from build123d import *

# Parameters (mm, degrees)
SKETCH1_R           = 1.4605
BOSS_EXTRUDE1_DEPTH = 3.175
CUT_EXTRUDE1_REACH  = 105.107
CUT_EXTRUDE2_REACH  = 105.107
SKETCH4_W           = 25.4
SKETCH4_H           = 7.62
CUT_EXTRUDE3_DEPTH  = 36.774302562


with BuildPart() as part:
    # Sketch1 → Boss-Extrude1 (new body)
    with BuildSketch(Plane.XY):
        with BuildLine():
            Line((0, 7.62), (0, 25.4))
            ThreePointArc((0, 25.4), (-17.960512242, -17.960512242), (25.4, 0))
            Line((25.4, 0), (16.51, 0))
            Line((16.51, 0), (16.51, -3.175))
            Line((16.51, -3.175), (13.589, -3.175))
            Line((13.589, -3.175), (13.589, -9.779))
            Line((13.589, -9.779), (15.494, -9.779))
            Line((15.494, -9.779), (15.494, -12.827))
            Line((15.494, -12.827), (13.589, -12.827))
            Line((13.589, -12.827), (10.541, -12.827))
            Line((10.541, -12.827), (8.636, -12.827))
            Line((8.636, -12.827), (8.636, -9.779))
            Line((8.636, -9.779), (10.541, -9.779))
            Line((10.541, -9.779), (10.541, -3.175))
            Line((10.541, -3.175), (7.62, -3.175))
            Line((7.62, -3.175), (7.62, 0))
            ThreePointArc((7.62, 0), (5.388153673, 5.388153673), (0, 7.62))
        make_face()
        with Locations((20.955, -1.5875)):
            Circle(SKETCH1_R, mode=Mode.SUBTRACT)
        Polygon((3.175, 1.833087105), (3.175, -1.833087105), (0, -3.666174209), (-3.175, -1.833087105), (-3.175, 1.833087105), (0, 3.666174209), align=None, mode=Mode.SUBTRACT)
    extrude(amount=BOSS_EXTRUDE1_DEPTH)

    # Sketch2 → Cut-Extrude1 (cut, up to next)
    with BuildSketch(Plane(origin=(0, 0, -93.472), x_dir=(-1, 0, 0), z_dir=(0, 0, -1)), mode=Mode.PRIVATE) as cut_extrude1_sk1:
        Polygon((-4.538711403, -7.782479393), (27.834438784, -7.782479393), (16.089332095, -38.12601526), (-4.538711403, -36.427419359), align=None)
    cut_extrude1_tool1 = extrude(cut_extrude1_sk1.sketch, amount=-CUT_EXTRUDE1_REACH, mode=Mode.PRIVATE) & part.part
    add(cut_extrude1_tool1.solids().sort_by_distance((-9.075281, -21.483297, -93.472))[0], mode=Mode.SUBTRACT)

    # Sketch3 → Cut-Extrude2 (cut, up to next)
    with BuildSketch(Plane(origin=(0, 0, -93.472), x_dir=(-1, 0, 0), z_dir=(0, 0, -1)), mode=Mode.PRIVATE) as cut_extrude2_sk1:
        Polygon((8.30871298, -7.782479393), (8.30871298, 15.866972004), (0, 15.866972004), (0, 32.212276886), (53.906645957, 11.420627768), (19.587788586, -19.264211479), align=None)
    cut_extrude2_tool1 = extrude(cut_extrude2_sk1.sketch, amount=-CUT_EXTRUDE2_REACH, mode=Mode.PRIVATE) & part.part
    add(cut_extrude2_tool1.solids().sort_by_distance((-22.758535, 7.548852, -93.472))[0], mode=Mode.SUBTRACT)

    # Sketch4 → Cut-Extrude3 (cut, through all)
    with BuildSketch(Plane(origin=(0, 0, 0), x_dir=(-1, 0, 0), z_dir=(0, 0, -1))):
        with Locations((-17.238711403, -21.181200427)):
            Rectangle(SKETCH4_W, SKETCH4_H)
    extrude(amount=-CUT_EXTRUDE3_DEPTH, mode=Mode.SUBTRACT)


solid = part.part
Design review of the part built by this model. Coordinates are the model's own, in mm. A direction names the side the tool comes from. Round coordinates to 2 decimals unless told otherwise and drop trailing zeros. Write each loop counter-clockwise with the first axis right and the second up, starting at its lowest first coordinate (ties: lowest second). Pieces come first, ordered by that corner, then holes. Notation, with made-up numbers: (-0.5, 22) -> (47.5, 22) arc R19 cw to (47.5, 29) -> close; hole circle Ø6 at (33, 49.5). An arc over 180 degrees is marked (long way). One line per item, written item: value. Start each with the question number.
Q1. Add section B-B (y = -11.5). Give the boundary of the cut face in (x, z) (3 decimals).
Q2. Add section C-C (z = 1.55). Give the boundary of the cut face in (x, y) (1 decimal), then the cut area to 3 significant figures.
Q3. Add section A-A (x = 9.5). Give the boundary of the cut face in (y, z) (3 decimals), then the cut area to 3 significant figures.
Q4. Insertion check: P1, Ø1, axis at x = 1, z = 1, coming from the -Y side; P2, Ø1.5, axis at y = -11, z = 2.5, coming from the -X side; P3, Ø1.5, axis at x = 15, z = 1, coming from the +Y side (3 decimals). Each pin has a flat end and moves straight along its axis. Give the tip position at first contact, or say it passes through.
Q5. Add section D-D (x = 13). Give the boundary of the cut face in (y, z) (3 decimals), then the cut area to 3 significant figures.
Q6. Tool access review of faces 4 (the face through (10.541, -7, 2)), 5 (the face through (3.175, 0, 2)), 6 (the face through (22, 0, 2)): name each direction out of +Z, -Z, +X, -X, +Y, -Y from which nothing blocks a thin tool from reaching the whole face with its end or side.
Q7. To check wall thickness, follow probe 1 along X at (y, z) = (-1.5, 2.6) (3 decimals); probe 2 along X at (y, z) = (-1, 1.85) (3 decimals); probe 3 along Y at (x, z) = (15, 2.4) (3 decimals). State the ranges of each line that lie inside material, in increasing order.
Q8. The part is to be moulded in two halves that separate along X. For faces 1 (the face through (12, -12.827, 2)), 2 (the face through (-8.309, 4, 2)), 3 (the face through (8, -4, 0)), say which applies: pulls with the +X half, pulls with the -X half, needs draft (parallel to the pull), parting line crosses it, or undercut.
Response:
1. outline: (4.539, 0) -> (8.636, 0) -> (8.636, 3.175) -> (4.539, 3.175) -> close; (15.494, 0) -> (22.648, 0) -> (22.648, 3.175) -> (15.494, 3.175) -> close
2. outline: (-8.3, -7.8) -> (4.5, -7.8) -> (4.5, -17.4) -> (18.5, -17.4) arc R25.4 ccw to (25.4, 0) -> (16.5, 0) -> (16.5, -3.2) -> (13.6, -3.2) -> (13.6, -9.8) -> (15.5, -9.8) -> (15.5, -12.8) -> (8.6, -12.8) -> (8.6, -9.8) -> (10.5, -9.8) -> (10.5, -3.2) -> (7.6, -3.2) -> (7.6, 0) arc R7.6 ccw to (0, 7.6) -> (0, 15.9) -> (-8.3, 15.9) -> close; hole (-3.2, -1.8) -> (0, -3.7) -> (3.2, -1.8) -> (3.2, 1.8) -> (0, 3.7) -> (-3.2, 1.8) -> close; hole circle Ø2.9 at (21, -1.6)
2. area: 492 mm^2
3. outline: (-17.371, 0) -> (-12.827, 0) -> (-12.827, 3.175) -> (-17.371, 3.175) -> close; (-9.779, 0) -> (-3.175, 0) -> (-3.175, 3.175) -> (-9.779, 3.175) -> close
3. area: 35.4 mm^2
4. P1: stops at y = -7.78
4. P2: stops at x = 4.54
4. P3: stops at y = -3.175
5. outline: (-17.371, 0) -> (-12.827, 0) -> (-12.827, 3.175) -> (-17.371, 3.175) -> close
5. area: 14.4 mm^2
6. face 4: +Z, -Z, +Y
6. face 5: +Z, -Z
6. face 6: +Z, -Z, +X, +Y
7. probe 1: x = -8.309 to -3.175, 3.175 to 7.62, 16.51 to 19.497, 22.413 to 25.356
7. probe 2: x = -8.309 to -3.175, 3.175 to 7.62, 16.51 to 19.618, 22.292 to 25.38
7. probe 3: y = -17.371 to -12.827, -9.779 to -3.175
8. face 1: undercut
8. face 2: pulls with the -X half
8. face 3: needs draft
